Check sheet for the modelled part. Datum: model origin and axes. Units: mm. A direction names the side the tool comes from. Coordinates: 2 decimals unless noted, no trailing zeros. Write each loop counter-clockwise with the first axis right and the second up, starting at its lowest first coordinate (ties: lowest second). Pieces come first, ordered by that corner, then holes. Notation, with made-up numbers: (85.25, 10) - (143.25, 10) arc R27 ccw to (143.25, 30) - close; hole circle Ø7 at (29.25, 66). An arc over 180 degrees is marked (long way). Write each question's results on one line, items separated by ' | '.
from build123d import *

# Parameters (mm, degrees)
SKETCH_R        = 9
PAD_DEPTH       = 226
SKETCH001_W     = 15
SKETCH001_H     = 8
PAD001_DEPTH    = 25
SKETCH002_R     = 4.1
POCKET_DEPTH    = 13.001
SKETCH003_R     = 4
POCKET001_DEPTH = 185


with BuildPart() as part:
    # Sketch → Pad (new body)
    with BuildSketch(Plane.XZ):
        Circle(SKETCH_R)
    extrude(amount=PAD_DEPTH)

    # Sketch001 (on Face2 of Pad) → Pad001 (join)
    with BuildSketch(Plane(origin=(0, 0, 0), x_dir=(1, 0, 0), z_dir=(0, 1, 0))):
        Rectangle(SKETCH001_W, SKETCH001_H)
    extrude(amount=PAD001_DEPTH)

    # Sketch002 (on Face6 of Pad001) → Pocket (cut, through all)
    with BuildSketch(Plane(origin=(0, 0, 4), x_dir=(-1, 0, 0), z_dir=(0, 0, 1))):
        with Locations((0, -17)):
            Circle(SKETCH002_R)
        with BuildLine():
            ThreePointArc((-8, -17), (0, -25), (8, -17))
            Line((8, -26), (8, -17))
            Line((-8, -26), (8, -26))
            Line((-8, -17), (-8, -26))
        make_face()
    extrude(amount=-POCKET_DEPTH, mode=Mode.SUBTRACT)

    # Sketch003 (on Face3 of Pocket) → Pocket001 (cut)
    with BuildSketch(Plane.XZ.offset(226)):
        Circle(SKETCH003_R)
    extrude(amount=-POCKET001_DEPTH, mode=Mode.SUBTRACT)


solid = part.part
1. Go/stop test with flat-tipped pins: pin 1 (4.5 mm diameter, centred on x = 0.5, y = 6.5, fed in from +Z); pin 2 (9 mm diameter, centred on x = -1.5, z = 0, fed in from -Y); pin 3 (9 mm diameter, centred on y = 11.5, z = 1, fed in from +X); pin 4 (2.5 mm diameter, centred on y = 14.5, z = 0.5, fed in from -X). Record where each tip stops, or that it passes through.
Values follow:
pin 1: stops at z = 4 | pin 2: stops at y = -226 | pin 3: stops at x = 7.5 | pin 4: stops at x = -7.5
2. Sectioned sample at B-B (z = 0). Record the cut outline in (x, y).
Values follow:
outline: (-9, -226) - (-4, -226) - (-4, -41) - (4, -41) - (4, -226) - (9, -226) - (9, 0) - (7.5, 0) - (7.5, 19.78) arc R8 ccw to (-7.5, 19.78) - (-7.5, 0) - (-9, 0) - close; hole circle Ø8.2 at (0, 17)
3. Draft check along X on faces 1 (the flat face through (0, 10, 4)), 2 (the cylindrical face through (-0.867, -134.795, -3.905)), 3 (the flat face through (-7.5, 10, 0)), 4 (the flat face through (7.5, 10, 0)). Enter one of: pulls with the +X half, pulls with the -X half, needs draft (parallel to the pull), parting line crosses it, or undercut.
Values follow:
face 1: needs draft | face 2: undercut | face 3: pulls with the -X half | face 4: pulls with the +X half
4. Sectioned sample at D-D (y = -63.5). Record the cut outline in (x, z).
Values follow:
outline: circle Ø18 at (0, 0); hole circle Ø8 at (0, 0)
5. Material ranges on L1, parallel to X at y = 17, z = 2.25; L2, parallel to Z at x = 0, y = -124.5; L3, parallel to X at y = -141.5, z = 0.25, recorded low to high. Write a range as [from, to].
Values follow:
L1: x = [-7.5, -4.1], [4.1, 7.5] | L2: z = [-9, -4], [4, 9] | L3: x = [-9, -3.99], [3.99, 9]
6. Sectioned sample at C-C (x = 0). Record the cut outline in (y, z), then the cut area to 3 significant figures.
Values follow:
outline: (-226, -9) - (0, -9) - (0, -4) - (12.9, -4) - (12.9, 4) - (0, 4) - (0, 9) - (-226, 9) - (-226, 4) - (-41, 4) - (-41, -4) - (-226, -4) - close; (21.1, -4) - (25, -4) - (25, 4) - (21.1, 4) - close | area: 2,720 mm^2
7. Access from +Z, -Z, +X, -X, +Y, -Y to the whole of each face (thin tool, end or side, straight path). Record for faces 5 (the flat face through (0, -41, 0)), 6 (the cylindrical face through (0, 25, 0)), 7 (the flat face through (0, 10, -4)).
Values follow:
face 5: -Y | face 6: +Z, -Z, +Y | face 7: -Z, +X, -X, +Y
8. Sectioned sample at A-A (y = 17). Record the cut outline in (x, z), then the cut area to 3 significant figures.
Values follow:
outline: (-7.5, -4) - (-4.1, -4) - (-4.1, 4) - (-7.5, 4) - close; (4.1, -4) - (7.5, -4) - (7.5, 4) - (4.1, 4) - close | area: 54.4 mm^2
